Read the model definition and answer for the solid it produces. Units are mm, in the model's axes. Coordinates: 2 decimals unless noted, no trailing zeros. Use one line per item in the form item = value.
from build123d import *

# Parameters (mm, degrees)
BOSS_EXTRUDE1_DEPTH = 1.5875
SKETCH2_R           = 6.35
SKETCH2_R_2         = 3.175
CUT_EXTRUDE1_DEPTH  = 316.731983488
SKETCH3_W           = 329.065813824
SKETCH3_H           = 177.30262506
CUT_EXTRUDE2_DEPTH  = 316.731983488
FILLET1_DEPTH       = 1.5875
SKETCH4_R           = 2.032
CUT_EXTRUDE3_DEPTH  = 2.54
SKETCH5_R           = 2.127
CUT_EXTRUDE4_DEPTH  = 2.54


with BuildPart() as part:
    # Sketch1 → Boss-Extrude1 (new body)
    with BuildSketch(Plane.XY):
        with BuildLine():
            add(Edge.make_bspline(
                [(0.000560351, 0.000130087), (0.810633127, 7.359196055), (8.649092025, 17.856605174), (26.286719818, 29.975176328), (52.111128271, 42.069215275), (89.597618475, 49.290763054), (131.400792109, 47.884831915), (173.256699242, 40.041104278), (217.961060472, 29.612974894), (256.952064401, 19.528920948), (290.35983767, 8.71099439), (301.273197721, 4.382828139), (314.816918223, -0.516206742), (309.846313895, 0.000130087)],
                knots=[0, 0, 0, 0, 0.060863618, 0.113688265, 0.188608742, 0.312908923, 0.448482434, 0.557612135, 0.691544113, 0.852438279, 0.92975597, 0.976058229, 1, 1, 1, 1], degree=3))
            add(Edge.make_bspline(
                [(309.846313895, 0.000130087), (303.956832565, 1.47095521), (293.989507544, 2.093987313), (276.26402299, 4.514356704), (260.846344817, 5.427413394), (235.858814759, 7.870306192), (205.101424636, 8.838080282), (157.718638092, 9.030650149), (110.497331172, 6.181495223), (66.506197185, -0.586669107), (36.454672816, -6.098499901), (15.316603331, -6.189065841), (1.230714189, -6.924076091), (0.000560351, 0.000130087)],
                knots=[0, 0, 0, 0, 0.057787081, 0.095274891, 0.171021118, 0.205339302, 0.335319146, 0.464904334, 0.658702312, 0.785511947, 0.893517288, 0.94309214, 1, 1, 1, 1], degree=3))
        make_face()
    extrude(amount=BOSS_EXTRUDE1_DEPTH)

    # Sketch2 → Cut-Extrude1 (cut, through all)
    with BuildSketch(Plane.XY.offset(1.5875)):
        with Locations((20.32, 10.16)):
            Circle(SKETCH2_R)
        with Locations((227.296313895, 19.050130087)):
            Circle(SKETCH2_R_2)
    extrude(amount=-CUT_EXTRUDE1_DEPTH, mode=Mode.SUBTRACT)

    # Sketch3 → Cut-Extrude2 (cut, through all)
    with BuildSketch(Plane.XY.offset(1.5875)):
        with Locations((74.193406983, 18.895182109)):
            Rectangle(SKETCH3_W, SKETCH3_H)
    extrude(amount=-CUT_EXTRUDE2_DEPTH, mode=Mode.SUBTRACT)

    # Fillet1: read off the stored shape, not the designer's step
    # Fillet1 outline → Fillet1 (cut)
    with BuildSketch(Plane.XY):
        with BuildLine():
            ThreePointArc((245.711534403, 6.855899952), (240.78695405, 9.238088014), (238.727660088, 14.306186276))
            ThreePointArc((238.727660088, 14.306186276), (241.790276652, 20.270898068), (248.380487069, 21.506427765))
            add(Edge.make_bspline(
                [(248.380487069, 21.506427765), (245.14201846, 22.403497776), (241.927955434, 23.272784833), (238.726313893, 24.121097226)],
                knots=[0.203822749, 0.203822749, 0.203822749, 0.203822749, 0.233593651, 0.233593651, 0.233593651, 0.233593651], degree=3))
            Line((238.726313893, 24.121097226), (238.726313894, 7.379528673))
            add(Edge.make_bspline(
                [(238.726313894, 7.379528673), (241.056196666, 7.224072569), (243.384717208, 7.05041014), (245.711534403, 6.855899952)],
                knots=[0.772010011, 0.772010011, 0.772010011, 0.772010011, 0.794337025, 0.794337025, 0.794337025, 0.794337025], degree=3))
        make_face()
    extrude(amount=FILLET1_DEPTH, mode=Mode.SUBTRACT)

    # Sketch4 → Cut-Extrude3 (cut)
    with BuildSketch(Plane.XY.offset(1.5875)):
        with Locations((246.346313895, 14.162958592)):
            Circle(SKETCH4_R)
    extrude(amount=-CUT_EXTRUDE3_DEPTH, mode=Mode.SUBTRACT)

    # Sketch5 → Cut-Extrude4 (cut)
    with BuildSketch(Plane.XY.offset(1.5875)):
        with Locations((260.720225155, 15.178172845)):
            Circle(SKETCH5_R)
        with Locations((283.157187456, 5.977798132)):
            Circle(SKETCH5_R)
    extrude(amount=-CUT_EXTRUDE4_DEPTH, mode=Mode.SUBTRACT)


solid = part.part
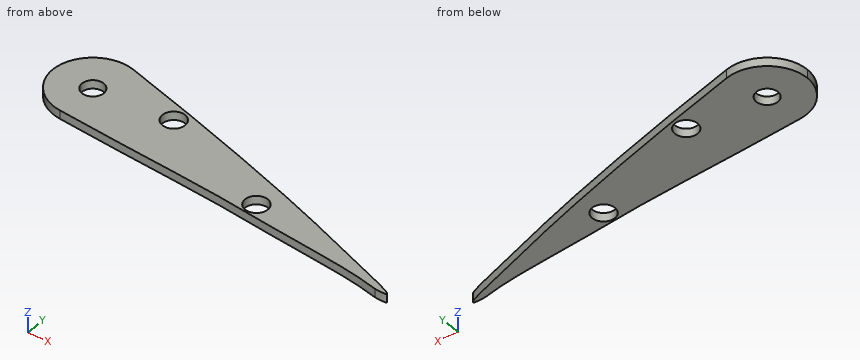
Item 1: This flat-tipped pin is pushed along its axis until it touches: P1, Ø3.5, axis at x = 283.16, y = 5.98, coming from the -Z side. Where does it stop, or does it pass through?
Results below:
P1 = through
Item 2: Find the intervals of material crossed by L1, parallel to Y at x = 245, z = 1.1; L2, parallel to Y at x = 292, z = 0.75; L3, parallel to Y at x = 294, z = 0.25, in increasing order.
Results below:
L1 = 6.95 to 12.64, 15.68 to 21.66
L2 = 2.48 to 7.92
L3 = 2.28 to 7.18
Item 3: The part is cut by section A-A on z = 1.25. Count the separate pieces of the cut face and the enclosed holes in it, plus the area to 3 significant figures.
Results below:
separate_pieces = 1
enclosed_holes = 3
area = 585 mm²
